Geometry check sheet. Reference: drawing and pictorial views, mm from the part's lowest x, y, z. A direction names the side the tool comes from. Give positions to 0.01 mm unless a question says otherwise; leave off trailing zeros. Write each loop counter-clockwise with the first axis right and the second up, starting at its lowest first coordinate (ties: lowest second). Pieces come first, ordered by that corner, then holes. Notation, with made-up numbers: (-15, 64) -> (4, 64) arc R35 cw to (4, 98) -> close; hole circle Ø10 at (-29, -4.75). An arc over 180 degrees is marked (long way). Use a Markdown table: item, result. Add a question column.
1. Cross-section at B-B (x = 22.5). Enter the section's corners in (y, z).
2. Cross-section at C-C (y = 42). Enter the section's corners in (x, z), then the cut area to 3 significant figures.
3. Set-up check for the marked faces 4, 5, 6, 7 and 8: record each of +Z, -Z, +X, -X, +Y, -Y from which the full face is reachable in a straight line by a thin tool's end or side.
4. Release check for a two-part mould opening along Z. For the marked faces 1, 2 and 3 record: released by +Z, released by -Z, zero draft, split by the parting line, or undercut.
5. Cross-section at D-D (x = 115.5). Enter the section's corners in (y, z).
6. Gauge pin test, flat ends, axial feed: P1, Ø1.5, axis at x = 61, y = 11, coming from the -Z side; P2, Ø22, axis at x = 103.5, y = 26, coming from the +Z side. Record the tip position at first contact, or that the pin passes through.
7. Scan lines: probe 1 along Z at (x, y) = (51.5, 31); probe 2 along X at (y, z) = (46.5, 32); probe 3 along Z at (x, y) = (48.5, 71). Record each from-to range of solid material in increasing order. Write a range as [from, to].
8. Cross-section at A-A (z = 32.5). Enter the section's corners in (x, y).
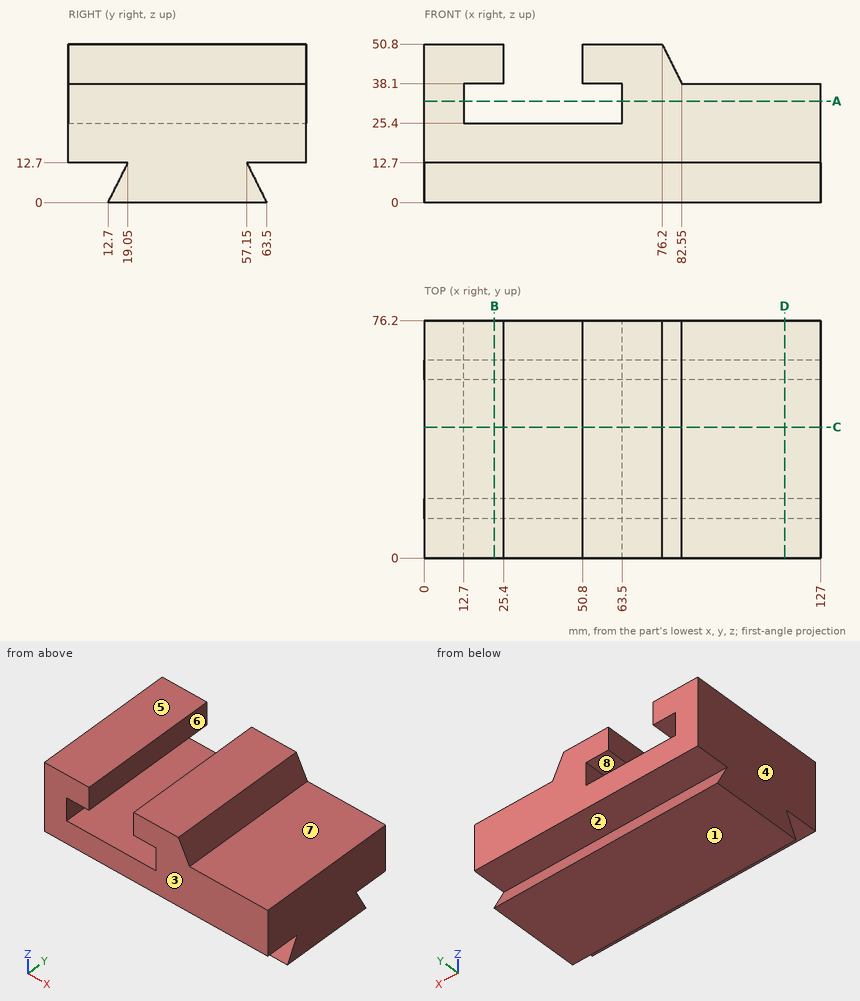
Worked answers:
| question | item | result |
|---|---|---|
| 1 | outline | (0, 12.7) -> (19.05, 12.7) -> (12.7, 0) -> (63.5, 0) -> (57.15, 12.7) -> (76.2, 12.7) -> (76.2, 25.4) -> (0, 25.4) -> close; (0, 38.1) -> (76.2, 38.1) -> (76.2, 50.8) -> (0, 50.8) -> close |
| 2 | outline | (0, 0) -> (127, 0) -> (127, 38.1) -> (82.55, 38.1) -> (76.2, 50.8) -> (50.8, 50.8) -> (50.8, 38.1) -> (63.5, 38.1) -> (63.5, 25.4) -> (12.7, 25.4) -> (12.7, 38.1) -> (25.4, 38.1) -> (25.4, 50.8) -> (0, 50.8) -> close |
| 2 | area | 4,880 mm² |
| 3 | face 4 | +Z, -Z, -X, +Y, -Y |
| 3 | face 5 | +Z, +X, -X, +Y, -Y |
| 3 | face 6 | +Z, +Y, -Y |
| 3 | face 7 | +Z, +X, +Y, -Y |
| 3 | face 8 | +Y, -Y |
| 4 | face 1 | released by -Z |
| 4 | face 2 | undercut |
| 4 | face 3 | zero draft |
| 5 | outline | (0, 12.7) -> (19.05, 12.7) -> (12.7, 0) -> (63.5, 0) -> (57.15, 12.7) -> (76.2, 12.7) -> (76.2, 38.1) -> (0, 38.1) -> close |
| 6 | P1 | stops at z = 12.7 |
| 6 | P2 | stops at z = 38.1 |
| 7 | probe 1 | z = [0, 25.4], [38.1, 50.8] |
| 7 | probe 2 | x = [0, 12.7], [63.5, 127] |
| 7 | probe 3 | z = [12.7, 25.4] |
| 8 | outline | (0, 0) -> (12.7, 0) -> (12.7, 76.2) -> (0, 76.2) -> close; (63.5, 0) -> (127, 0) -> (127, 76.2) -> (63.5, 76.2) -> close |
